Source: CAD feature listing. Evaluate the final solid. Frame: model axes, mm. Face numbers are marked on the shaded views. A direction names the side the tool comes from. Give positions to 0.01 mm unless a question says otherwise; leave off trailing zeros. Write each loop counter-clockwise with the first axis right and the second up, starting at its lowest first coordinate (ties: lowest second). Pieces come first, ordered by that corner, then holes. Notation, with made-up numbers: M 7,-23.75 L 37,-23.75 A21 ccw 37,-19.75 Z; hole C -5.75,72 d7. An arc over 180 degrees is marked long. Use CSV: the item, a comma, the result in double quotes. Start each with the question number.
from build123d import *

# Parameters (mm, degrees)
SKETCH1_W           = 40
SKETCH1_H           = 20
BOSS_EXTRUDE1_DEPTH = 9.5
FILLET1_START       = -21
FILLET1_DEPTH       = 41
FILLET1_START_2     = -11
FILLET1_2_DEPTH     = 22
SKETCH4_R           = 7.5
BOSS_EXTRUDE2_DEPTH = 8
SKETCH5_R           = 2.15
CUT_EXTRUDE1_DEPTH  = 34.260336859
SKETCH6_R           = 7.65
BOSS_EXTRUDE3_DEPTH = 8


with BuildPart() as part:
    # Sketch1 → Boss-Extrude1 (new body)
    with BuildSketch(Plane.XY):
        Rectangle(SKETCH1_W, SKETCH1_H)
    extrude(amount=BOSS_EXTRUDE1_DEPTH)

    # Fillet1: read off the stored shape, not the designer's step
    # Fillet1 outline → Fillet1 (cut)
    with BuildSketch(Plane.YZ.offset(FILLET1_START)):
        with BuildLine():
            Line((10, 9.5), (9, 9.5))
            add(Edge.make_bspline(
                [(9, 9.5), (10, 9.5), (10, 8.5)],
                knots=[0, 0, 0, 1, 1, 1], degree=2, weights=[1, 0.707106781, 1]))
            Line((10, 8.5), (10, 9.5))
        make_face()
        with BuildLine():
            add(Edge.make_bspline(
                [(-9, 9.5), (-10, 9.5), (-10, 8.5)],
                knots=[0, 0, 0, 1, 1, 1], degree=2, weights=[1, 0.707106781, 1]))
            Line((-9, 9.5), (-10, 9.5))
            Line((-10, 9.5), (-10, 8.5))
        make_face()
    extrude(amount=FILLET1_DEPTH, mode=Mode.SUBTRACT)

    # Fillet1 2 outline → Fillet1 2 (cut)
    with BuildSketch(Plane(origin=(0, 0, 0), x_dir=(1, 0, 0), z_dir=(0, 1, 0)).offset(FILLET1_START_2)):
        with BuildLine():
            Line((-20, -9.5), (-19, -9.5))
            add(Edge.make_bspline(
                [(-19, -9.5), (-20, -9.5), (-20, -8.5)],
                knots=[0, 0, 0, 1, 1, 1], degree=2, weights=[1, 0.707106781, 1]))
            Line((-20, -8.5), (-20, -9.5))
        make_face()
        with BuildLine():
            add(Edge.make_bspline(
                [(19, -9.5), (20, -9.5), (20, -8.5)],
                knots=[0, 0, 0, 1, 1, 1], degree=2, weights=[1, 0.707106781, 1]))
            Line((19, -9.5), (20, -9.5))
            Line((20, -9.5), (20, -8.5))
        make_face()
    extrude(amount=FILLET1_2_DEPTH, mode=Mode.SUBTRACT)

    # Sketch4 → Boss-Extrude2 (add)
    with BuildSketch(Plane.XY.offset(9.5)):
        with Locations((-10.628602575, 0)):
            Circle(SKETCH4_R)
    extrude(amount=BOSS_EXTRUDE2_DEPTH)

    # Sketch5 → Cut-Extrude1 (cut, through all)
    with BuildSketch(Plane.XZ.offset(10)):
        with Locations(Location((-15.628602575, 4.7, 0), (0, 0, 270))):
            Circle(SKETCH5_R)
        with Locations(Location((-5.628602575, 4.7, 0), (0, 0, 270))):
            Circle(SKETCH5_R)
        with Locations(Location((5.5, 4.7, 0), (0, 0, 270))):
            Circle(SKETCH5_R)
        with Locations(Location((15.5, 4.7, 0), (0, 0, 270))):
            Circle(SKETCH5_R)
    extrude(amount=-CUT_EXTRUDE1_DEPTH, mode=Mode.SUBTRACT)

    # Sketch6 → Boss-Extrude3 (add)
    with BuildSketch(Plane.XY.offset(9.5)):
        with Locations((-10.628602575, 0)):
            Circle(SKETCH6_R)
    extrude(amount=BOSS_EXTRUDE3_DEPTH)


solid = part.part
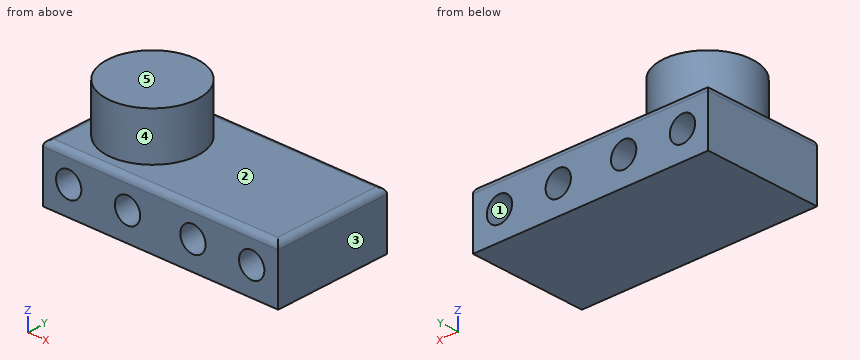
1. Section A-A on z = 4.7. Return loops of the section in (x, y).
2. Access query for the marked faces 4 and 5. Directions: +Z, -Z, +X, -X, +Y, -Y. A direction counts if a zero-diameter tool reaches every point of the face in a straight line with its end or side. Return the directions, or none.
3. First-contact query: pin 1 (8 mm diameter, centred on x = -11, y = 4, fed in from -Z); pin 2 (1.5 mm diameter, centred on x = 13, y = 3.5, fed in from +Z). Flat tips, straight axial feed; report the tip coordinate or a pass-through.
4. Section C-C on y = 5.5. Give the number of separate pieces and of enclosed holes in the cut face, then the cut area to 3 significant figures.
5. Section B-B on z = 11.5. Return loops of the section in (x, y), then the cut area to 3 significant figures.
6. Line query: probe 1 along X at (y, z) = (-2.75, 4.7); probe 2 along Z at (x, y) = (-5.5, 1); probe 3 along X at (y, z) = (-3, 4.25). Output: solid intervals per line, ascending.
7. Pull-direction query (X, two-part tool) for the marked faces 1, 2 and 3; classes: released by +X, released by -X, zero draft, split by the parting line, or undercut.
Resolved:
1,outline,"M -20,-10 L -17.78,-10 L -17.78,10 L -20,10 Z; M -13.48,-10 L -7.78,-10 L -7.78,10 L -13.48,10 Z; M -3.48,-10 L 3.35,-10 L 3.35,10 L -3.48,10 Z; M 7.65,-10 L 13.35,-10 L 13.35,10 L 7.65,10 Z; M 17.65,-10 L 20,-10 L 20,10 L 17.65,10 Z"
2,face 4,"+Z"
2,face 5,"+Z, +X, -X, +Y, -Y"
3,pin 1,"stops at z = 0"
3,pin 2,"stops at z = 9.5"
4,separate pieces,"1"
4,enclosed holes,"4"
4,area,"407 mm2"
5,outline,"C -10.63,0 d15.3"
5,area,"184 mm2"
6,probe 1,"x = -20 to -17.78, -13.48 to -7.78, -3.48 to 3.35, 7.65 to 13.35, 17.65 to 20"
6,probe 2,"z = 0 to 2.55, 6.85 to 17.5"
6,probe 3,"x = -20 to -17.73, -13.53 to -7.73, -3.53 to 3.4, 7.6 to 13.4, 17.6 to 20"
7,face 1,"undercut"
7,face 2,"zero draft"
7,face 3,"released by +X"
